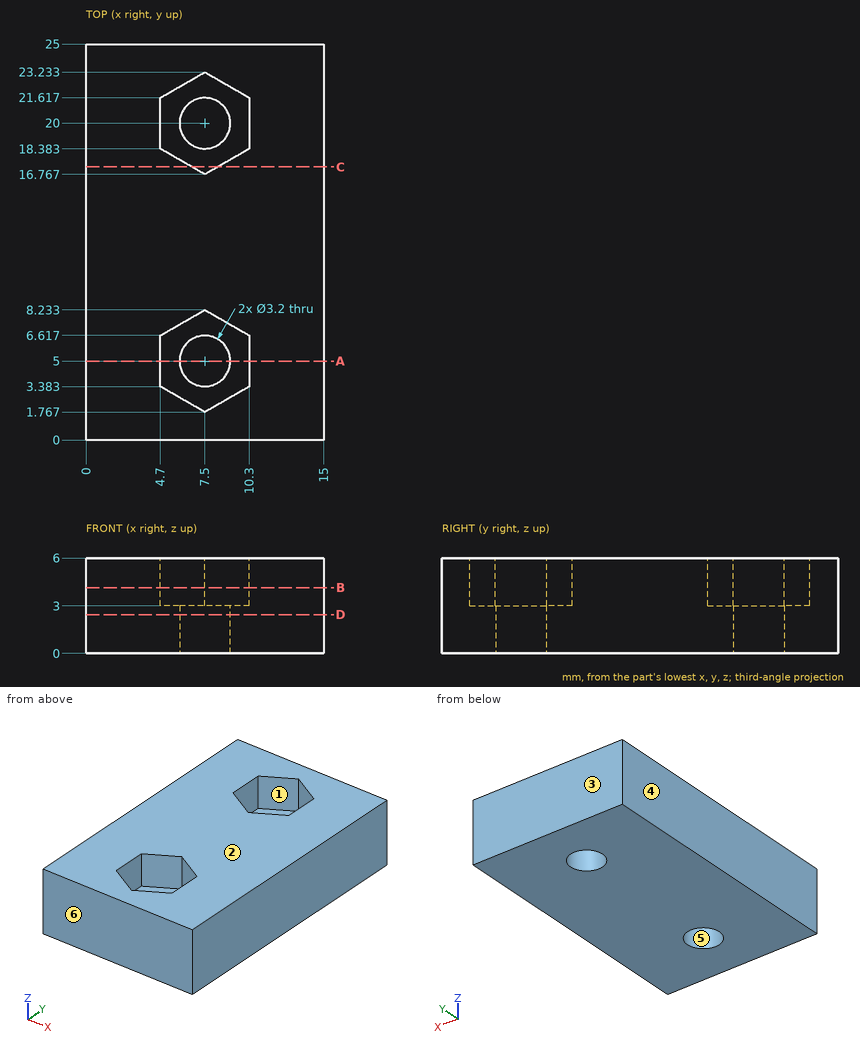
Part print with two shaded views. Sizes in mm from the minimum x, y, z corner. A direction names the side the tool comes from. Coordinates: 2 decimals unless noted, no trailing zeros. Order: outer loops, then holes, each group sorted by start corner. A loop starts at its lowest first (then second) coordinate and runs counter-clockwise, first axis right, second up.
(1) Which spindle directions (+Z, -Z, +X, -X, +Y, -Y) get a long thin tool onto all of the face, cutting with end or side? Do the marked faces 1 and 2. Say none if no direction does.
Solution:
face 1: +Z
face 2: +Z, +X, -X, +Y, -Y
(2) Drill centre lines: L1, parallel to Y at x = 7.5, z = 1; L2, parallel to Y at x = 5.75, z = 4.2; L3, parallel to X at y = 20.25, z = 0.4. Where is each one in solid material? Low to high.
Solution:
L1: y = 0 to 3.4, 6.6 to 18.4, 21.6 to 25
L2: y = 0 to 2.78, 7.22 to 17.78, 22.22 to 25
L3: x = 0 to 5.92, 9.08 to 15
(3) Saw through at D-D, the plane z = 2.45. Write the cut outline in (x, y), and give its area (3 significant figures).
Solution:
outline: (0, 0) - (15, 0) - (15, 25) - (0, 25) - close; hole circle Ø3.2 at (7.5, 5); hole circle Ø3.2 at (7.5, 20)
area: 359 mm2
(4) Pin check, flat tip, straight feed: pin 1 Ø1.7 at (x, y) = (8, 6.5) entering from +Z. Stop position of the tip, or through.
Solution:
pin 1: stops at z = 3
(5) Saw through at A-A, the plane y = 5. Write the cut outline in (x, z).
Solution:
outline: (0, 0) - (5.9, 0) - (5.9, 3) - (4.7, 3) - (4.7, 6) - (0, 6) - close; (9.1, 0) - (15, 0) - (15, 6) - (10.3, 6) - (10.3, 3) - (9.1, 3) - close
(6) Saw through at C-C, the plane y = 17.25. Write the cut outline in (x, z).
Solution:
outline: (0, 0) - (15, 0) - (15, 6) - (8.34, 6) - (8.34, 3) - (6.66, 3) - (6.66, 6) - (0, 6) - close
(7) Saw through at B-B, the plane z = 4.15. Write the cut outline in (x, y).
Solution:
outline: (0, 0) - (15, 0) - (15, 25) - (0, 25) - close; hole (4.7, 3.38) - (7.5, 1.77) - (10.3, 3.38) - (10.3, 6.62) - (7.5, 8.23) - (4.7, 6.62) - close; hole (4.7, 18.38) - (7.5, 16.77) - (10.3, 18.38) - (10.3, 21.62) - (7.5, 23.23) - (4.7, 21.62) - close
(8) Mould opens along Y. For the marked faces 3, 4, 5 and 6 say: released by +Y, released by -Y, zero draft, split by the parting line, or undercut.
Solution:
face 3: released by +Y
face 4: zero draft
face 5: undercut
face 6: released by -Y
